Input: part model. Units: mm. Frame: model coordinates. A direction names the side the tool comes from. Round coordinates to 2 decimals unless told otherwise and drop trailing zeros. Loops run counter-clockwise (first coordinate to the right, second up) from the corner with the lowest first, then second, coordinate; pieces in that order, holes last. Notation, with made-up numbers: (-21, 3) - (38, 3) arc R18 ccw to (38, 32) - close; hole circle Ø10 at (-34.75, 0.5). An arc over 180 degrees is marked (long way). One line per question, with ' | ' between items. Start each with the question number.
from build123d import *

# Parameters (mm, degrees)
EXTRUDE_1_DEPTH     = 8
SKETCH_2_R          = 4
EXTRUDE_2_DEPTH     = 19.5
EXTRUDE_3_DEPTH     = 3
SKETCH_4_R          = 5
EXTRUDE_4_DEPTH     = 12
EXTRUDE_5_DEPTH     = 2
SKETCH_10_R         = 6.937077861
EXTRUDE_6_DEPTH     = 18
EXTRUDE_6_TAPER     = -5
SKETCH_11_R         = 4.303815727
CUT_EXTRUDE_2_DEPTH = 18
SKETCH_12_R         = 1.731234863
CUT_EXTRUDE_3_DEPTH = 8
FILLET_1_R          = 2
SKETCH_13_R         = 0.923714742
CUT_EXTRUDE_4_DEPTH = 63.5


with BuildPart() as part:
    # 草图1 → 凸台-拉伸1 (new body)
    with BuildSketch(Plane.XY):
        Polygon((-3.698048527, 5.858706094), (-6.922812574, -0.273250922), (-3.224764047, -6.131957016), (3.698048527, -5.858706094), (6.922812574, 0.273250922), (3.224764047, 6.131957016), align=None)
    extrude(amount=EXTRUDE_1_DEPTH)

    # 草图2 → 凸台-拉伸2 (add)
    with BuildSketch(Plane(origin=(0, 0, 0), x_dir=(-1, 0, 0), z_dir=(0, 0, -1))):
        Circle(SKETCH_2_R)
    extrude(amount=EXTRUDE_2_DEPTH)

    # 草图3 → 凸台-拉伸3 (add)
    with BuildSketch(Plane(origin=(0, 0, -19.5), x_dir=(-1, 0, 0), z_dir=(0, 0, -1))):
        Polygon((4.007714345, 5.941327246), (-3.141483154, 6.441446057), (-7.149197499, 0.500118811), (-4.007714345, -5.941327246), (3.141483154, -6.441446057), (7.149197499, -0.500118811), align=None)
    extrude(amount=EXTRUDE_3_DEPTH)

    # 草图4 → 凸台-拉伸4 (add)
    with BuildSketch(Plane(origin=(0, 0, -22.5), x_dir=(-1, 0, 0), z_dir=(0, 0, -1))):
        Circle(SKETCH_4_R)
    extrude(amount=EXTRUDE_4_DEPTH)

    # 草图5 → 凸台-拉伸5 (add)
    with BuildSketch(Plane(origin=(0, 0, -34.5), x_dir=(-1, 0, 0), z_dir=(0, 0, -1))):
        Polygon((1.187065622, 1.98096152), (-1.122030189, 2.018509744), (-2.309095811, 0.037548225), (-1.187065622, -1.98096152), (1.122030189, -2.018509744), (2.309095811, -0.037548225), align=None)
    extrude(amount=EXTRUDE_5_DEPTH)

    # 草图10 → 凸台-拉伸6 (add)
    with BuildSketch(Plane.XY.offset(8)):
        Circle(SKETCH_10_R)
    extrude(amount=EXTRUDE_6_DEPTH, taper=EXTRUDE_6_TAPER)

    # 草图11 → 切除-拉伸2 (cut)
    with BuildSketch(Plane.XY.offset(26)):
        Circle(SKETCH_11_R)
    extrude(amount=-CUT_EXTRUDE_2_DEPTH, mode=Mode.SUBTRACT)

    # 草图12 → 切除-拉伸3 (cut)
    with BuildSketch(Plane.XY.offset(8)):
        Circle(SKETCH_12_R)
    extrude(amount=-CUT_EXTRUDE_3_DEPTH, mode=Mode.SUBTRACT)

    # 圆角1
    fillet_1_edges = [part.edges().sort_by_distance(p)[0] for p in [
        (-8.511873804, 0, 26),
        (-4.303815727, 0, 26),
    ]]
    fillet(fillet_1_edges, radius=FILLET_1_R)

    # 草图13 → 切除-拉伸4 (cut, through all)
    with BuildSketch(Plane(origin=(0, 0, -36.5), x_dir=(-1, 0, 0), z_dir=(0, 0, -1))):
        Circle(SKETCH_13_R)
    extrude(amount=-CUT_EXTRUDE_4_DEPTH, mode=Mode.SUBTRACT)


solid = part.part
(1) Section B-B, the plane z = -28. Output: boundary loops of the cut face in (x, y).
(2) Line query: line 1 along Y through (x, z) = (0, -11); line 2 along Z through (x, y) = (-0.75, -5.75); line 3 along Z through (x, y) = (1, -1). Output: solid intervals per line, ascending. Write a range as from..to.
(3) Pin query (flat end, axial travel): P1, Ø5, axis at y = -4, z = -25.5, coming from the +X side; P2, Ø6, axis at y = -4.5, z = 1.5, coming from the -X side; P3, Ø1.7, axis at x = -0.5, y = -0.5, coming from the +Z side. Return the tip coordinate at first contact, or that it passes through.
(4) Section C-C, the plane z = 19. Output: boundary loops of the cut face in (x, y).
(5) Reachability of faces 1 (the face through (0.48, -6.19, -20.98)), 2 (the face through (-5.1, -3.16, 3.94)), 3 (the face through (-5.288, 2.836, 3.944)), 4 (the face through (5.288, -2.836, 3.944)) from +Z, -Z, +X, -X, +Y, -Y: full face, straight path, thin tool, end or side. Return the list, or none.
(6) Section A-A, the plane z = 2.5. Output: boundary loops of the cut face in (x, y), plus the area to 3 significant figures.
(7) Pull-direction query (Z, two-part tool) for faces 5 (the face through (5.1, 3.16, 3.94)), 6 (the face through (-3.415, -2.619, 16.112)), 7 (the face through (-1, 0.5, -36.5)); classes: released by +Z, released by -Z, zero draft, split by the parting line, or undercut.
Derived:
1) outline: circle Ø10 at (0, 0); hole circle Ø1.85 at (0, 0)
2) line 1: y = -4..-0.92, 0.92..4 | line 2: z = -22.5..-19.5, 0..25.94 | line 3: z = -36.5..0
3) P1: stops at x = 4.77 | P2: stops at x = -6.15 | P3: stops at z = 0
4) outline: circle Ø15.8 at (0, 0); hole circle Ø8.61 at (0, 0)
5) face 1: -Z, +X, -Y | face 2: -X, -Y | face 3: -X, +Y | face 4: +X, -Y
6) outline: (-6.92, -0.27) - (-3.22, -6.13) - (3.7, -5.86) - (6.92, 0.27) - (3.22, 6.13) - (-3.7, 5.86) - close; hole circle Ø3.46 at (0, 0) | area: 115 mm²
7) face 5: undercut | face 6: zero draft | face 7: released by -Z
